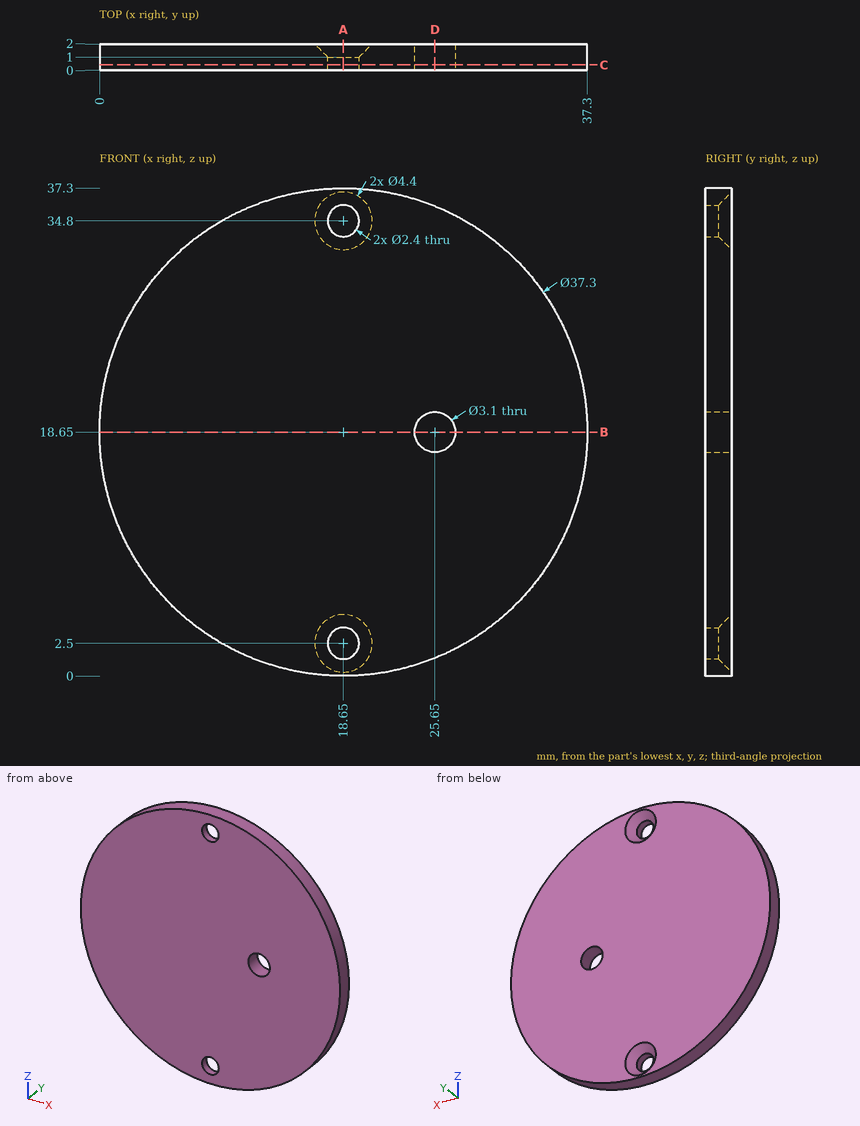
Answer from the drawing. Dimensions are ordinates in mm from the lowest x, y and z of the part. Give positions to 0.01 mm unless a question says otherwise; leave off trailing zeros. Loops run counter-clockwise (first coordinate to the right, second up) from the corner with the lowest first, then second, coordinate; pieces in that order, holes last. Notation, with made-up numbers: (22, 4.25) - (50, 4.25) arc R18 cw to (50, 9.25) - close; hole circle Ø10 at (-6, 89.5). An arc over 180 degrees is marked (long way). Answer as a JSON object with one key per item and string values.
1. A cutting plane is placed at C-C (y = 0.4). Write down the section's boundary in (x, z).
Determined:
{"outline": "circle Ø37.3 at (18.65, 18.65); hole circle Ø2.4 at (18.65, 2.5); hole circle Ø2.4 at (18.65, 34.8); hole circle Ø3.1 at (25.65, 18.65)"}
2. A cutting plane is placed at A-A (x = 18.65). Write down the section's boundary in (y, z).
Determined:
{"outline": "(0, 0) - (2, 0) - (2, 0.3) - (1, 1.3) - (0, 1.3) - close; (0, 3.7) - (1, 3.7) - (2, 4.7) - (2, 32.6) - (1, 33.6) - (0, 33.6) - close; (0, 36) - (1, 36) - (2, 37) - (2, 37.3) - (0, 37.3) - close"}
3. Find the intervals of material crossed by L1, parallel to Z at x = 18.65, y = 0.5; L2, parallel to Z at x = 25.65, y = 1.1; L3, parallel to X at y = 0.75, z = 34.8, in increasing order. Write a range as [from, to].
Determined:
{"L1": "[0, 1.3], [3.7, 33.6], [36, 37.3]", "L2": "[1.36, 17.1], [20.2, 35.94]", "L3": "[9.32, 17.45], [19.85, 27.98]"}
4. A cutting plane is placed at D-D (x = 25.65). Write down the section's boundary in (y, z), then the cut area to 3 significant figures.
Determined:
{"outline": "(0, 1.36) - (2, 1.36) - (2, 17.1) - (0, 17.1) - close; (0, 20.2) - (2, 20.2) - (2, 35.94) - (0, 35.94) - close", "area": "62.9 mm²"}
5. A flat-ended cylindrical pin translates along its axis: pin 1 Ø3.5 at (x, z) = (25.65, 18.65) entering from -Y. Find the tip coordinate at first contact, or state that the pin passes through.
Determined:
{"pin 1": "y = 0"}
6. A cutting plane is placed at B-B (z = 18.65). Write down the section's boundary in (x, y).
Determined:
{"outline": "(0, 0) - (24.1, 0) - (24.1, 2) - (0, 2) - close; (27.2, 0) - (37.3, 0) - (37.3, 2) - (27.2, 2) - close"}
